```python
from build123d import *

# Parameters (mm, degrees)
F1_DEPTH = 4.5
F0_R     = 1.9
F2_DEPTH = 1.27
F3_SIZE  = 0.508
F4_W     = 0.7
F4_H     = 0.6
F5_DEPTH = 13.5
F6_SIZE  = 0.2032


with BuildPart() as f1:
    # F0 (on Top) → F1 (new body)
    with BuildSketch(Plane.XY):
        with BuildLine():
            Line((5.1, -2.006139996), (5.1, 1.3))
            Line((5.1, 1.3), (-5.1, 1.3))
            Line((-5.1, 1.3), (-5.1, -2.006139996))
            ThreePointArc((-5.1, -2.006139996), (-3.4965183315, -3.6096216645), (-5.1, -5.213103333))
            Line((-5.1, -5.213103333), (-5.1, -7.7))
            Line((-5.1, -7.7), (5.1, -7.7))
            Line((5.1, -7.7), (5.1, -5.213103333))
            ThreePointArc((5.1, -5.213103333), (3.4965183315, -3.6096216645), (5.1, -2.006139996))
        make_face()
    extrude(amount=F1_DEPTH)

    # F0 (on Top) → F2 (join)
    with BuildSketch(Plane.XY):
        Polygon((5.1, 5.6912479922), (3.4809927456, 7.7), (-3.4809927456, 7.7), (-5.1, 5.6912479922), (-5.1, 1.3), (5.1, 1.3), align=None)
        with Locations((0, 4.5)):
            Circle(F0_R, mode=Mode.SUBTRACT)
        with BuildLine():
            ThreePointArc((-5.1, -5.213103333), (-3.4965183315, -3.6096216645), (-5.1, -2.006139996))
            Line((-5.1, -2.006139996), (-5.1, -5.213103333))
        make_face()
        with BuildLine():
            Line((5.1, -5.213103333), (5.1, -2.006139996))
            ThreePointArc((5.1, -2.006139996), (3.4965183315, -3.6096216645), (5.1, -5.213103333))
        make_face()
    extrude(amount=F2_DEPTH)

    # F3
    f3_edges = [f1.edges().sort_by_distance(p)[0] for p in [
        (-5.1, -6.456552, 4.5),
        (0, 1.3, 4.5),
        (5.1, -0.35307, 4.5),
        (3.496518, -3.609622, 4.5),
        (-3.496518, -3.609622, 4.5),
        (5.1, -6.456552, 4.5),
        (-5.1, -0.35307, 4.5),
    ]]
    chamfer(f3_edges, length=F3_SIZE)

    # F4 (on face) → F5 (join)
    with BuildSketch(Plane.XZ.offset(7.7)):
        with Locations((-2.55, 2.8)):
            Rectangle(F4_W, F4_H)
        with Locations((0, 2.8)):
            Rectangle(F4_W, F4_H)
        with Locations((2.55, 2.8)):
            Rectangle(F4_W, F4_H)
    extrude(amount=F5_DEPTH)

    # F6
    f6_edges = [f1.edges().sort_by_distance(p)[0] for p in [
        (-2.55, -21.2, 3.1),
        (-2.9, -21.2, 2.8),
        (-2.55, -21.2, 2.5),
        (-2.2, -21.2, 2.8),
        (0, -21.2, 3.1),
        (-0.35, -21.2, 2.8),
        (0, -21.2, 2.5),
        (0.35, -21.2, 2.8),
        (2.55, -21.2, 3.1),
        (2.2, -21.2, 2.8),
        (2.55, -21.2, 2.5),
        (2.9, -21.2, 2.8),
    ]]
    chamfer(f6_edges, length=F6_SIZE)


solid = f1.part
```
Verification items for the finished model (mm, model axes). A direction names the side the tool comes from. Give positions to 0.01 mm unless a question says otherwise; leave off trailing zeros. Loops run counter-clockwise (first coordinate to the right, second up) from the corner with the lowest first, then second, coordinate; pieces in that order, holes last.
1. Mould release check, pull along X, two halves, no side actions. Record for faces 4 (the conical face through (3.36, -3.65, 4.13)), 5 (the cylindrical face through (-0.247, 6.384, 0.626)), 6 (the flat face through (0, 1.3, 3)): released by +X, released by -X, zero draft, split by the parting line, or undercut.
2. Section check B-B, the plane x = 1.5. Enter the section's corners in (y, z).
3. Set-up check for faces 1 (the cylindrical face through (-3.497, -3.574, 2.612)), 2 (the flat face through (0, 2, 1.27)), 3 (the flat face through (4, -4, 1.27)): record each of +Z, -Z, +X, -X, +Y, -Y from which the full face is reachable in a straight line by a thin tool's end or side.
4. Section check A-A, the plane y = 4.5. Enter the section's corners in (x, z).
5. Go/stop test with flat-tipped pins: pin 1 Ø0.6 at (x, y) = (2.5, -15) entering from +Z; pin 2 Ø0.6 at (x, y) = (0, -14.5) entering from -Z; pin 3 Ø1.3 at (x, y) = (-4.5, -3) entering from +Z. Record where each tip stops, or that it passes through.
6. Thickness scan on line 1 (Y direction, x = 0, z = 0.85); line 2 (Y direction, x = -2.5, z = 1.55); line 3 (Y direction, x = 0.5, z = 1.2). Record the ranges inside material, lowest first.
7. Section check C-C, the plane x = -1.25. Enter the section's corners in (y, z).
Geometry says:
1. face 4: released by +X
1. face 5: undercut
1. face 6: zero draft
2. outline: (-7.7, 0) - (3.33, 0) - (3.33, 1.27) - (1.3, 1.27) - (1.3, 3.99) - (0.79, 4.5) - (-7.7, 4.5) - close; (5.67, 0) - (7.7, 0) - (7.7, 1.27) - (5.67, 1.27) - close
3. face 1: +Z, -X
3. face 2: +Z, +X, -X, +Y
3. face 3: +Z, +X
4. outline: (-5.1, 0) - (-1.9, 0) - (-1.9, 1.27) - (-5.1, 1.27) - close; (1.9, 0) - (5.1, 0) - (5.1, 1.27) - (1.9, 1.27) - close
5. pin 1: stops at z = 3.1
5. pin 2: stops at z = 2.5
5. pin 3: stops at z = 1.27
6. line 1: y = -7.7 to 2.6, 6.4 to 7.7
6. line 2: y = -7.7 to 1.3
6. line 3: y = -7.7 to 2.67, 6.33 to 7.7
7. outline: (-7.7, 0) - (3.07, 0) - (3.07, 1.27) - (1.3, 1.27) - (1.3, 3.99) - (0.79, 4.5) - (-7.7, 4.5) - close; (5.93, 0) - (7.7, 0) - (7.7, 1.27) - (5.93, 1.27) - close
